Can you work these out from the drawing? Everything is in mm from the part's minimum corner. A direction names the side the tool comes from. Coordinates: 2 decimals unless noted, no trailing zeros. Loops run counter-clockwise (first coordinate to the right, second up) from the corner with the lowest first, then second, coordinate; pieces in that order, holes last. Notation, with made-up numbers: (-12, 15.25) -> (29, 15.25) arc R9 ccw to (29, 30.25) -> close; hole circle Ø9 at (11.5, 62). An arc over 180 degrees is marked (long way). Use one line per item in the form item = value. Start each with the question number.
(1) Imagine slicing it at B-B (y = 5.5). List the corners of the cut face in (x, z) for me.
(2) Imagine slicing it at D-D (x = 2). List the corners of the cut face in (y, z) for me.
(3) I need wall thicknesses on line 1 (Z direction, x = 0.75, y = 4.5); line 2 (Z direction, x = 4.25, y = 2.75); line 3 (Y direction, x = 7.25, z = 1.5). Which ranges of each line are inside material? Lowest first, please. Write a range as [from, to].
(4) On a 3-axis mill with a long thin cutter (end or side, diameter ignored), from which of +Z, -Z, +X, -X, +Y, -Y can I reach the whole of each face in a straight line? I mean the marked faces 1, 2 and 3. Say none if no direction works.
(5) Imagine slicing it at C-C (z = 12). List the corners of the cut face in (x, y) for me.
(6) Imagine slicing it at A-A (x = 7.5). List the corners of the cut face in (y, z) for me, plus the area to 3 significant figures.
(7) I'm going to push flat-ended pins straight in: pin 1 (5 mm diameter, centred on y = 3, z = 2.5, fed in from -X); pin 2 (2 mm diameter, centred on x = 9, z = 12, fed in from +Y); pin 3 (1.5 mm diameter, centred on x = 12, z = 15.5, fed in from -Y) (1 decimal). Where does each tip first touch, or does it pass through?
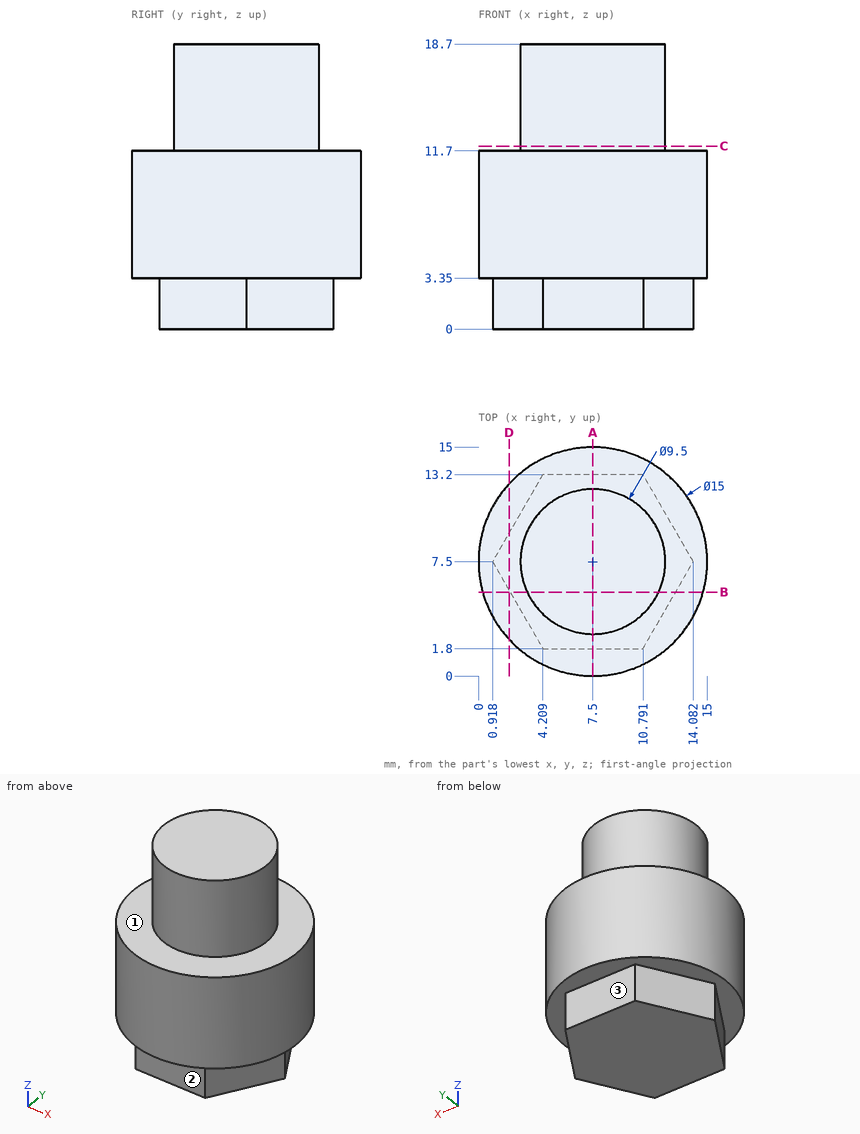
Worked out:
q1.outline = (0.27, 3.35) -> (2.07, 3.35) -> (2.07, 0) -> (12.93, 0) -> (12.93, 3.35) -> (14.73, 3.35) -> (14.73, 11.7) -> (11.81, 11.7) -> (11.81, 18.7) -> (3.19, 18.7) -> (3.19, 11.7) -> (0.27, 11.7) -> close
q2.outline = (2.4, 3.35) -> (5.63, 3.35) -> (5.63, 0) -> (9.37, 0) -> (9.37, 3.35) -> (12.6, 3.35) -> (12.6, 11.7) -> (2.4, 11.7) -> close
q3.line_1 = [3.35, 11.7]
q3.line_2 = [0, 11.7]
q3.line_3 = [1.8, 13.2]
q4.face_1 = +Z
q4.face_2 = -Z, +X, -X, -Y
q4.face_3 = -Z, +X, -X, +Y
q5.outline = circle Ø9.5 at (7.5, 7.5)
q6.outline = (0, 3.35) -> (1.8, 3.35) -> (1.8, 0) -> (13.2, 0) -> (13.2, 3.35) -> (15, 3.35) -> (15, 11.7) -> (12.25, 11.7) -> (12.25, 18.7) -> (2.75, 18.7) -> (2.75, 11.7) -> (0, 11.7) -> close
q6.area = 230 mm2
q7.pin_1 = 0.31
q7.pin_2 = 14.98
q7.pin_3 = 4.6
